from build123d import *

# Parameters (mm, degrees)
SKETCH1_W             = 21.4
SKETCH1_H             = 53.2
BOSS_EXTRUDE1_DEPTH   = 2
SKETCH2_W             = 21.4
SKETCH2_H             = 13.7
BOSS_EXTRUDE2_DEPTH   = 11.3
SKETCH3_R             = 3.65
CUT_EXTRUDE1_DEPTH    = 4
F_2_0MM_DOWEL_HOLE1_D = 2
BOSS_EXTRUDE3_DEPTH   = 1
BOSS_EXTRUDE4_DEPTH   = 5


with BuildPart() as part:
    # Sketch1 → Boss-Extrude1 (new body)
    with BuildSketch(Plane(origin=(0, 0, 0), x_dir=(1, 0, 0), z_dir=(0, 1, 0))):
        with Locations((10.7, 26.6)):
            Rectangle(SKETCH1_W, SKETCH1_H)
    extrude(amount=BOSS_EXTRUDE1_DEPTH)

    # Sketch2 → Boss-Extrude2 (add)
    with BuildSketch(Plane(origin=(0, 2, 0), x_dir=(1, 0, 0), z_dir=(0, 1, 0))):
        with Locations((10.7, 46.35)):
            Rectangle(SKETCH2_W, SKETCH2_H)
    extrude(amount=BOSS_EXTRUDE2_DEPTH)

    # Sketch3 → Cut-Extrude1 (cut)
    with BuildSketch(Plane(origin=(0, 0, -53.2), x_dir=(-1, 0, 0), z_dir=(0, 0, -1))):
        with Locations((-10.7, 7.65)):
            Circle(SKETCH3_R)
    extrude(amount=-CUT_EXTRUDE1_DEPTH, mode=Mode.SUBTRACT)

    # Ø2.0mm Dowel Hole1 (through all)
    with Locations(Plane(origin=(0, 2, 0), x_dir=(1, 0, 0), z_dir=(0, 1, 0))):
        with Locations((2.45, 36.869115366), (18.95, 36.869115366), (18.95, 1.869115366), (2.45, 1.869115366)):
            Hole(F_2_0MM_DOWEL_HOLE1_D / 2)



with BuildPart() as body_2:
    # Sketch10 → Boss-Extrude3 (new body)
    with BuildSketch(Plane.XY):
        with BuildLine():
            Line((7.05, 0), (14.35, 0))
            ThreePointArc((14.35, 0), (14.526776695, -0.073223305), (14.6, -0.25))
            Line((14.6, -0.25), (14.6, -2.65))
            ThreePointArc((14.6, -2.65), (14.526776695, -2.826776695), (14.35, -2.9))
            Line((14.35, -2.9), (7.05, -2.9))
            ThreePointArc((7.05, -2.9), (6.873223305, -2.826776695), (6.8, -2.65))
            Line((6.8, -2.65), (6.8, -0.25))
            ThreePointArc((6.8, -0.25), (6.873223305, -0.073223305), (7.05, 0))
        make_face()
    extrude(amount=BOSS_EXTRUDE3_DEPTH)


with BuildPart() as part_1:
    add(part.part)

    add(body_2.part)  # Boss-Extrude4 merges body 2
    # Sketch10<2> → Boss-Extrude4 (add)
    with BuildSketch(Plane.XY):
        with BuildLine():
            Line((7.05, 0), (14.35, 0))
            ThreePointArc((14.35, 0), (14.526776695, -0.073223305), (14.6, -0.25))
            Line((14.6, -0.25), (14.6, -2.65))
            ThreePointArc((14.6, -2.65), (14.526776695, -2.826776695), (14.35, -2.9))
            Line((14.35, -2.9), (7.05, -2.9))
            ThreePointArc((7.05, -2.9), (6.873223305, -2.826776695), (6.8, -2.65))
            Line((6.8, -2.65), (6.8, -0.25))
            ThreePointArc((6.8, -0.25), (6.873223305, -0.073223305), (7.05, 0))
        make_face()
    extrude(amount=-BOSS_EXTRUDE4_DEPTH)


solid = part_1.part
Design review of the part built by this model. Coordinates are the model's own, in mm. A direction names the side the tool comes from. Round coordinates to 2 decimals unless told otherwise and drop trailing zeros. Write each loop counter-clockwise with the first axis right and the second up, starting at its lowest first coordinate (ties: lowest second). Pieces come first, ordered by that corner, then holes. Notation, with made-up numbers: M 86,-29.5 L 110,-29.5 A32 ccw 110,-3.5 Z; hole C 60.5,1 d3. An arc over 180 degrees is marked long. One line per item, written item: value. Start each with the question number.
1. To check wall thickness, follow probe 1 along Z at (x, y) = (2.45, 1.3); probe 2 along Y at (x, z) = (10.7, -51.35); probe 3 along Z at (x, y) = (4, 2.5). State the ranges of each line that lie inside material, in increasing order. Write a range as from..to.
2. Take a section at D-D on z = -34. State the section outline as (x, y) points, then the cut area to 3 significant figures.
3. Take a section at A-A on x = 18.95. State the section outline as (y, z) points, then the cut area to 3 significant figures.
4. Draft analysis for pull direction Y (two halves, no side actions). For faces 4 (the face through (11, -1, -5)), 5 (the face through (11, 8, -49.2)), 6 (the face through (10.6, 0, 0.5)), state which applies: pulls with the +Y half, pulls with the -Y half, needs draft (parallel to the pull), parting line crosses it, or undercut.
5. Take a section at B-B on y = 5.25. State the section outline as (x, z) points, then the cut area to 3 significant figures.
6. Clearance check with flat-ended pins moving along their axes: P1, Ø6, axis at x = 10.5, y = 9, coming from the -Z side; P2, Ø3, axis at x = 9, z = -47.5, coming from the -Y side; P3, Ø1.9, axis at y = -2, z = -2.5, coming from the -X side; P4, Ø1.5, axis at x = 11, y = -2, coming from the -Z side. State where each tip first meets the part, or that it passes through.
7. For faces 1 (the face through (14.6, -1, -2)), 2 (the face through (6.8, -1, -2)), 3 (the face through (11, 2, -20)), list the 3-axis set-ups (+Z, -Z, +X, -X, +Y, -Y) from which the entire face can be reached by the end or side of a thin tool; tool diameter is ignored.
8. Take a section at C-C on y = 7.65. State the section outline as (x, z) points.
Computed:
1. probe 1: z = -53.2..-37.87, -35.87..-2.87, -0.87..0
1. probe 2: y = 0..4, 11.3..13.3
1. probe 3: z = -53.2..-39.5
2. outline: M 0,0 L 21.4,0 L 21.4,2 L 0,2 Z
2. area: 42.8 mm²
3. outline: M 0,-53.2 L 13.3,-53.2 L 13.3,-39.5 L 2,-39.5 L 2,-37.87 L 0,-37.87 Z; M 0,-35.87 L 2,-35.87 L 2,-2.87 L 0,-2.87 Z; M 0,-0.87 L 2,-0.87 L 2,0 L 0,0 Z
3. area: 253 mm²
4. face 4: needs draft
4. face 5: undercut
4. face 6: pulls with the +Y half
5. outline: M 0,-53.2 L 7.95,-53.2 L 7.95,-49.2 L 13.45,-49.2 L 13.45,-53.2 L 21.4,-53.2 L 21.4,-39.5 L 0,-39.5 Z
5. area: 271 mm²
6. P1: stops at z = -53.2
6. P2: stops at y = 0
6. P3: stops at x = 6.8
6. P4: stops at z = -5
7. face 1: +Z, -Z, +X, -Y
7. face 2: +Z, -Z, -X, -Y
7. face 3: +Z, +X, -X, +Y
8. outline: M 0,-53.2 L 7.05,-53.2 L 7.05,-49.2 L 14.35,-49.2 L 14.35,-53.2 L 21.4,-53.2 L 21.4,-39.5 L 0,-39.5 Z
